from build123d import *

# Parameters (mm, degrees)
F0_R     = 3
F1_DEPTH = 2
F2_R     = 4
F3_DEPTH = 2
F5_W     = 6
F5_H     = 6
F6_DEPTH = 25
F7_D     = 5
F7_DEPTH = 2.5
F7_TIP   = 1.5021515476


with BuildPart() as f1:
    # F0 (on Top) → F1 (new body)
    with BuildSketch(Plane.XY):
        Circle(F0_R)
    extrude(amount=F1_DEPTH)

    # F2 (on face) → F3 (join)
    with BuildSketch(Plane.XY.offset(2)):
        Circle(F2_R)
    extrude(amount=F3_DEPTH)

    # F5 (on face) → F6 (intersect)
    with BuildSketch(Plane.XY.offset(4)):
        Rectangle(F5_W, F5_H)
    extrude(amount=-F6_DEPTH, mode=Mode.INTERSECT)

    # F7
    with Locations(Plane.XY.offset(4)):
        with Locations((0, 0)):
            Hole(F7_D / 2, depth=F7_DEPTH)
            with Locations((0, 0, -(F7_DEPTH + F7_TIP / 2))):  # 118° drill point
                Cone(0, F7_D / 2, F7_TIP, mode=Mode.SUBTRACT)


solid = f1.part
Input: part model. Units: mm. Frame: model coordinates. A direction names the side the tool comes from. Give positions to 0.01 mm unless a question says otherwise; leave off trailing zeros. Order: outer loops, then holes, each group sorted by start corner. A loop starts at its lowest first (then second) coordinate and runs counter-clockwise, first axis right, second up.
Q1. Ray query, probe 1 along X at (y, z) = (0, 2.75); probe 2 along Y at (x, z) = (2, 3). Return the intervals inside material, ascending.
Checked values:
probe 1: x = -3 to -2.5, 2.5 to 3
probe 2: y = -3 to -1.5, 1.5 to 3
Q2. Draft query along X for faces 5 (the flat face through (0, -3, 3)), 6 (the cylindrical face through (0.54, -2.44, 2.73)), 7 (the flat face through (3, 0, 3)). Return one class per face: +X half, -X half, draft (parallel to the pull), parting line (faces both ways), or undercut.
Checked values:
face 5: draft
face 6: undercut
face 7: +X half
Q3. Set-up query: faces 1 (the flat face through (-2.3, 2.4, 2)), 2 (the cylindrical face through (-3, 0, 1)), 3 (the flat face through (-2.3, -2.3, 2)), 4 (the flat face through (2.3, -2.4, 2)). Return all of +Z, -Z, +X, -X, +Y, -Y with unobstructed straight access to the full face (end or side cutting, diameter ignored); none if empty.
Checked values:
face 1: -Z, -X, +Y
face 2: -Z
face 3: -Z, -X, -Y
face 4: -Z, +X, -Y
Q4. Section A-A on z = 3. Output: boundary loops of the cut face in (x, y), and give its area (3 significant figures).
Checked values:
outline: (-3, -2.65) arc R4 ccw to (-2.65, -3) - (2.65, -3) arc R4 ccw to (3, -2.65) - (3, 2.65) arc R4 ccw to (2.65, 3) - (-2.65, 3) arc R4 ccw to (-3, 2.65) - close; hole circle Ø5 at (0, 0)
area: 16.1 mm2
Q5. Contact query for a flat-ended pin moving along its axis: pin 1 Ø3.5 at (x, y) = (-1.5, -1) entering from -Z. Output: stop coordinate, or through.
Checked values:
pin 1: stops at z = 0
